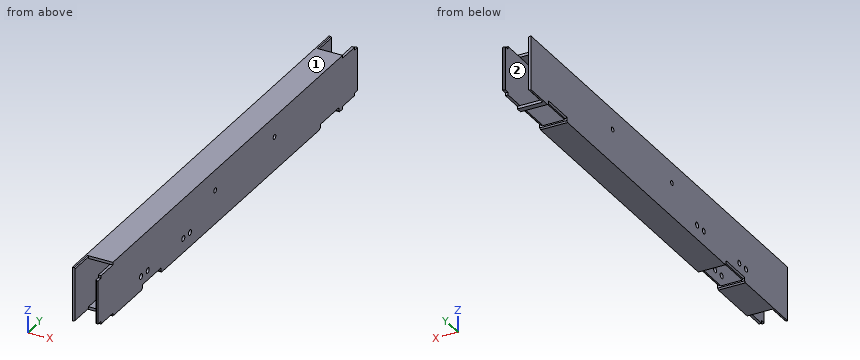
Solid Edge part; units mm, degrees
sketch "Sketch1" plane through (0, 0, 0) normal (0, -1, 0) x (1, 0, 0)
  line L0 (-16, -36) -> (16, -36)
  line L1 (16, -36) -> (16, 36)
  line L2 (16, 36) -> (-16, 36)
  line L3 (-16, 36) -> (-16, -36)
  line L4 (-20, -40) -> (20, -40)
  line L5 (20, -40) -> (20, 40)
  line L6 (20, 40) -> (-20, 40)
  line L7 (-20, 40) -> (-20, -40)
  dimension "D1" = 20
  dimension "D2" = 20
extrude "Protrusion1" add sketch "Sketch1" along normal mid plane 700
sketch "Sketch2" plane through (-20, 0, 0) normal (-1, 0, 0) x (0, -1, 0)
  line L0 (180.5, -40) -> (230.5, -40)
  line L1 (230.5, -40) -> (230.5, -35)
  line L2 (230.5, -35) -> (180.5, -35)
  line L3 (180.5, -35) -> (180.5, -40)
  line L4 (-299.5, -40) -> (-249.5, -40)
  line L5 (-249.5, -40) -> (-249.5, -35)
  line L6 (-249.5, -35) -> (-299.5, -35)
  line L7 (-299.5, -35) -> (-299.5, -40)
  dimension "D1" = 249.5
  dimension "D2" = 249.5
  dimension "D3" = 230.5
  dimension "D4" = 180.5
extrude "Cutout1" cut sketch "Sketch2" against normal through all
chamfer "Chamfer1" distance 2 angle 45 2 edges at (0, -230.5, -40) (0, -180.5, -40)
chamfer "Fase_5" distance 2 angle 45 2 edges at (0, 249.5, -40) (0, 299.5, -40)
chamfer "Fase_6" distance 2 angle 45 2 edges at (20, 274.5, -35) (-20, 274.5, -35)
chamfer "Fase_7" distance 2 angle 45 2 edges at (20, -205.5, -35) (-20, -205.5, -35)
sketch "Sketch3" plane through (20, 0, 0) normal (1, 0, 0) x (0, 1, 0)
  circle A0 centre (-216, -19) radius 4
  circle A1 centre (-120, -19) radius 4
  circle A2 centre (-102, -19) radius 4
  circle A3 centre (-234, -19) radius 4
  dimension "D1" = 120
  dimension "D2" = 234
  dimension "D3" = 216
  dimension "D4" = 234
extrude "Cutout2" cut sketch "Sketch3" against normal through all
sketch "Sketch4" plane through (-20, 0, 0) normal (-1, 0, 0) x (0, -1, 0)
  circle A0 centre (-126, 10) radius 3.5
  circle A1 centre (34, 10) radius 3.5
  dimension "D1" = 126
  dimension "D2" = 126
extrude "Cutout3" cut sketch "Sketch4" against normal through all
sketch "Sketch5" plane through (-20, -2, 0) normal (-1, 0, 0) x (0, -1, 0)
  line L0 (348, 40) -> (344, 40)
  line L1 (344, 40) -> (344, -40)
  line L2 (344, -40) -> (348, -40)
  line L3 (348, -40) -> (348, 40)
  dimension "D1" = 348
extrude "Cutout4" cut sketch "Sketch5" against normal up to vertex (36 mm away)
sketch "Sketch6" plane through (20, 0, 0) normal (1, 0, 0) x (0, 1, 0)
  line L0 (-350, 40) -> (-310, 40)
  line L1 (-310, 40) -> (-310, 36)
  line L2 (-310, 36) -> (-342, 36)
  line L3 (-342, 36) -> (-342, 32)
  line L4 (-342, 32) -> (-350, 32)
  line L5 (-350, 32) -> (-350, 40)
  dimension "D1" = 310
  dimension "D2" = 350
  dimension "D3" = 310
  dimension "D4" = 342
extrude "Cutout5" cut sketch "Sketch6" against normal blind 36
mirror "Mirror1" about plane through (0, 0, 0) normal (0, 0, 1) of "Cutout5"
mirror "Mirror2" about plane through (0, 0, 0) normal (0, -1, 0) of "Cutout4", "Cutout5", "Mirror1"
chamfer "Fase_11" distance 1.5 angle 45 4 edges at (-16, -328, 40) (-16, -328, -40) (-16, 328, 40) (-16, 328, -40)
chamfer "Fase_13" distance 1.5 angle 45 2 edges at (16, -350, 0) (16, 350, 0)
properties material "Aluminium, 6061-T6"
CAD build for the part. Positions are in the model's coordinates, mm. Face numbers are marked on the shaded views. A direction names the side the tool comes from. Coordinates: 2 decimals unless noted, no trailing zeros. Loops run counter-clockwise (first coordinate to the right, second up) from the corner with the lowest first, then second, coordinate; pieces in that order, holes last. Notation, with made-up numbers: (44.25, 59) - (48.25, 59) arc R13 cw to (48.25, 74) - close; hole circle Ø9 at (65, -2.5). An arc over 180 degrees is marked (long way). Use one line per item in the form item = value. Start each with the question number.
1) Flat gauge pins, fed straight in: pin 1 (1.2 mm diameter, centred on x = 19, y = 346.5, fed in from +Z); pin 2 (1.2 mm diameter, centred on x = 18, y = 320.5, fed in from -Z); pin 3 (2 mm diameter, centred on x = 18, z = -34, fed in from +Y). Where does each tip first touch, or does it go through?
2) Drill centre lines: L1, parallel to X at y = 154, z = -27.5; L2, parallel to Z at x = -17, y = 126; L3, parallel to Z at x = 12, y = 87. Where is each one in solid material? Low to high. Write a range as from..to.
3) Band-saw the part on B-B (x = 9). Give the cut face in (y, z).
4) Band-saw the part on C-C (y = 15). Give the cut face in (x, z).
5) Band-saw the part on A-A (z = 23). Give the cut face in (x, y).
6) Tool access for the marked faces 1 and 2: list every direction of +Z, -Z, +X, -X, +Y, -Y with a clear straight run to the whole face (end or side of a thin tool).
Check values:
q1.pin_1 = 32
q1.pin_2 = -36
q1.pin_3 = 342
q2.L1 = -20..-16, 16..20
q2.L2 = -40..6.5, 13.5..40
q2.L3 = -40..-36, 36..40
q3.outline = (-310, -40) - (-232.5, -40) - (-230.5, -38) - (-230.5, -36) - (-310, -36) - close; (-310, 36) - (310, 36) - (310, 40) - (-310, 40) - close; (-180.5, -38) - (-178.5, -40) - (247.5, -40) - (249.5, -38) - (249.5, -36) - (-180.5, -36) - close; (299.5, -38) - (301.5, -40) - (310, -40) - (310, -36) - (299.5, -36) - close
q4.outline = (-20, -40) - (20, -40) - (20, 40) - (-20, 40) - close; hole (-16, -36) - (16, -36) - (16, 36) - (-16, 36) - close
q5.outline = (-20, -346) - (-16, -346) - (-16, 346) - (-20, 346) - close; (16, -348.5) - (17.5, -350) - (20, -350) - (20, 350) - (17.5, 350) - (16, 348.5) - close
q6.face_1 = +Z, +X, -X, +Y, -Y
q6.face_2 = +Y, -Y
